Source: CAD feature listing. Evaluate the final solid. Frame: model axes, mm. Round coordinates to 2 decimals unless told otherwise and drop trailing zeros. Order: outer loops, then holes, each group sorted by start corner. A loop starts at its lowest first (then second) coordinate and runs counter-clockwise, first axis right, second up. Notation, with made-up numbers: M -17,29.25 L 24,29.25 A24 cw 24,42.25 Z; hole C 61,-38.75 d7. An arc over 180 degrees is marked long. Use CSV: the item, a comma, the result in double quotes. Start each with the question number.
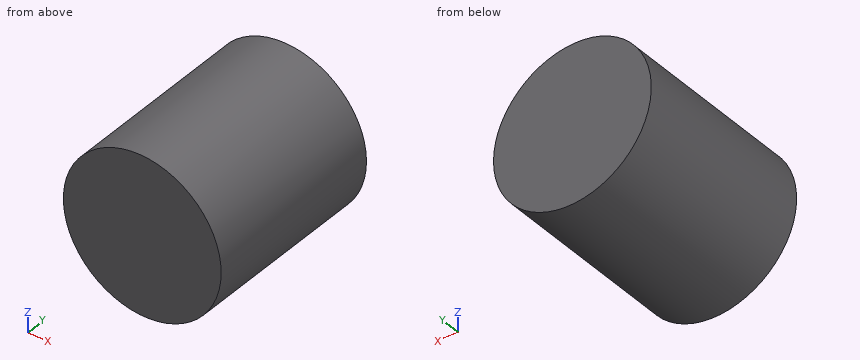
```python
from build123d import *

# Parameters (mm, degrees)
CROQUIS1_R                 = 63
SALIENTE_EXTRUIR1_DEPTH    = 145
CROQUIS2_R                 = 60
CORTAR_EXTRUIR1_DEPTH      = 2
CORTAR_EXTRUIR1_DEPTH_BACK = 142
CROQUIS3_R                 = 63
SALIENTE_EXTRUIR2_DEPTH    = 3


with BuildPart() as part:
    # Croquis1 → Saliente-Extruir1 (new body)
    with BuildSketch(Plane(origin=(0, 0, 0), x_dir=(1, 0, 0), z_dir=(0, 1, 0))):
        Circle(CROQUIS1_R)
    extrude(amount=SALIENTE_EXTRUIR1_DEPTH)

    # Croquis2 → Cortar-Extruir1 (cut, two sides)
    with BuildSketch(Plane(origin=(0, 145, 0), x_dir=(1, 0, 0), z_dir=(0, 1, 0))) as cortar_extruir1_sk:
        Circle(CROQUIS2_R)
    extrude(amount=CORTAR_EXTRUIR1_DEPTH, mode=Mode.SUBTRACT)
    extrude(cortar_extruir1_sk.sketch, amount=-CORTAR_EXTRUIR1_DEPTH_BACK, mode=Mode.SUBTRACT)

    # Croquis3 → Saliente-Extruir2 (add)
    with BuildSketch(Plane(origin=(0, 145, 0), x_dir=(1, 0, 0), z_dir=(0, 1, 0))):
        Circle(CROQUIS3_R)
    extrude(amount=SALIENTE_EXTRUIR2_DEPTH)


solid = part.part
```
(1) Section B-B on z = 0. Return loops of the section in (x, y), plus the area to 3 significant figures.
(2) Line query: line 1 along Y through (x, z) = (34, -45.5); line 2 along X through (y, z) = (83, 0). Output: solid intervals per line, ascending.
(3) Section C-C on y = 62.5. Return loops of the section in (x, z).
(4) Contact query for flat-ended pins moving along their axis: P1, Ø1.5, axis at x = 6, y = 69, coming from the -Z side; P2, Ø1, axis at y = 82.5, z = 10, coming from the +X side; P3, Ø1, axis at y = 20, z = 8.5, coming from the -X side. Output: stop coordinate, or through.
(5) Section A-A on x = 0. Return loops of the section in (y, z), plus the area to 3 significant figures.
Results below:
1,outline,"M -63,0 L 63,0 L 63,148 L -63,148 Z; hole M -60,3 L 60,3 L 60,145 L -60,145 Z"
1,area,"1,610 mm2"
2,line 1,"y = 0 to 3, 145 to 148"
2,line 2,"x = -63 to -60, 60 to 63"
3,outline,"C 0,0 d126; hole C 0,0 d120"
4,P1,"stops at z = -62.78"
4,P2,"stops at x = 62.28"
4,P3,"stops at x = -62.49"
5,outline,"M 0,-63 L 148,-63 L 148,63 L 0,63 Z; hole M 3,-60 L 145,-60 L 145,60 L 3,60 Z"
5,area,"1,610 mm2"
